from build123d import *

# Parameters (mm, degrees)
RESSALTO_EXTRUS_O1_DEPTH = 3
FILETE1_R                = 15
FILETE2_R                = 2


with BuildPart() as part:
    # Esboço1 → Ressalto-extrusão1 (new body)
    with BuildSketch(Plane.XY):
        Polygon((-23.5, 0), (-16.5, 0), (-16.5, 3), (16.5, 3), (16.5, 0), (23.5, 0), (23.5, 12), (3.5, 92), (1.5, 92), (1.5, 38), (-1.5, 38), (-1.5, 92), (-3.5, 92), (-23.5, 12), align=None)
    extrude(amount=RESSALTO_EXTRUS_O1_DEPTH)

    # Filete1
    filete1_edges = [part.edges().sort_by_distance(p)[0] for p in [
        (-23.5, 12, 1.5),
        (23.5, 12, 1.5),
    ]]
    fillet(filete1_edges, radius=FILETE1_R)

    # Filete2
    filete2_edges = [part.edges().sort_by_distance(p)[0] for p in [
        (-3.5, 92, 1.5),
        (3.5, 92, 1.5),
    ]]
    fillet(filete2_edges, radius=FILETE2_R)


solid = part.part
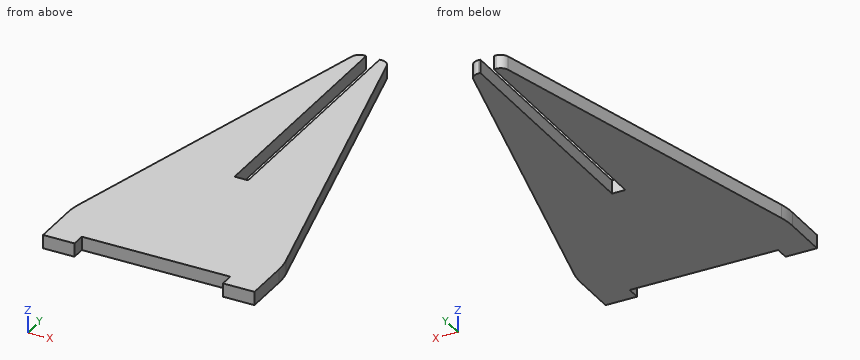
CAD build for the part. Positions are in the model's coordinates, mm. Coordinates: 2 decimals unless noted, no trailing zeros. Write each loop counter-clockwise with the first axis right and the second up, starting at its lowest first coordinate (ties: lowest second). Pieces come first, ordered by that corner, then holes. Notation, with made-up numbers: (27, 22) - (85, 22) arc R16 ccw to (85, 42) - close; hole circle Ø9 at (38.25, 57.5). An arc over 180 degrees is marked (long way). Use a Markdown table: item, result. Add a question column.
Item 1: Band-saw the part on B-B, the plane z = 0.7. Give the cut face in (x, y).
Item 2: Band-saw the part on D-D, the plane x = -12. Give the cut face in (y, z), and give its area (3 significant figures).
Item 3: Drill centre lines: L1, parallel to Y at x = -1, z = 2.5; L2, parallel to X at y = 55, z = 0.6; L3, parallel to X at y = 44, z = 1.65. Where is each one in solid material? Low to high. Write a range as from..to.
Item 4: Band-saw the part on A-A, the plane y = 59. Give the cut face in (x, z), and give its area (3 significant figures).
Item 5: Band-saw the part on C-C, the plane y = 41. Give the cut face in (x, z).
Item 6: Flat gauge pins, fed straight in: pin 1 (1.5 mm diameter, centred on x = -0.5, z = 1, fed in from +Y); pin 2 (1.5 mm diameter, centred on y = 73.5, z = 2, fed in from -X); pin 3 (10 mm diameter, centred on x = 0, y = 46.5, fed in from +Z); pin 4 (0.9 mm diameter, centred on y = 54, z = 1.5, fed in from +X). Where does each tip first touch, or does it go through?
Numbers:
| question | item | result |
|---|---|---|
| 1 | outline | (-23.5, 0) - (-16.5, 0) - (-16.5, 3) - (16.5, 3) - (16.5, 0) - (23.5, 0) - (23.5, 10.15) arc R15 ccw to (23.05, 13.79) - (3.88, 90.49) arc R2 ccw to (1.94, 92) - (1.5, 92) - (1.5, 38) - (-1.5, 38) - (-1.5, 92) - (-1.94, 92) arc R2 ccw to (-3.88, 90.49) - (-23.05, 13.79) arc R15 ccw to (-23.5, 10.15) - close |
| 2 | outline | (3, 0) - (58, 0) - (58, 3) - (3, 3) - close |
| 2 | area | 165 mm2 |
| 3 | L1 | 3..38 |
| 3 | L2 | -12.75..-1.5, 1.5..12.75 |
| 3 | L3 | -15.5..-1.5, 1.5..15.5 |
| 4 | outline | (-11.75, 0) - (-1.5, 0) - (-1.5, 3) - (-11.75, 3) - close; (1.5, 0) - (11.75, 0) - (11.75, 3) - (1.5, 3) - close |
| 4 | area | 61.5 mm2 |
| 5 | outline | (-16.25, 0) - (-1.5, 0) - (-1.5, 3) - (-16.25, 3) - close; (1.5, 0) - (16.25, 0) - (16.25, 3) - (1.5, 3) - close |
| 6 | pin 1 | y = 38 |
| 6 | pin 2 | x = -8.31 |
| 6 | pin 3 | z = 3 |
| 6 | pin 4 | x = 13.11 |
